Geometry check sheet. Reference: the model listing, model coordinates, mm. Round coordinates to 2 decimals unless told otherwise and drop trailing zeros. Write each loop counter-clockwise with the first axis right and the second up, starting at its lowest first coordinate (ties: lowest second). Pieces come first, ordered by that corner, then holes. Notation, with made-up numbers: (36.25, 69) - (84.25, 69) arc R8 ccw to (84.25, 81) - close; hole circle Ø3 at (69.25, -38.75). An arc over 180 degrees is marked (long way). Return JSON: item names as keys, results as strings.
```python
from build123d import *

# Parameters (mm, degrees)
SKETCH1_W                                  = 63.5
SKETCH1_H                                  = 30.48
BOSS_EXTRUDE1_DEPTH                        = 6.35
TAP_DRILL_FOR_8_32_TAP1_D                  = 3.4544
TAP_DRILL_FOR_8_32_TAP1_DEPTH              = 6.35
TAP_DRILL_FOR_8_32_TAP1_TIP                = 1.037806461
F_6_CLOSE_CLEARANCE_HOLE_COUNTERSINK_D     = 3.6576
F_6_CLOSE_CLEARANCE_HOLE_COUNTERSINK_DEPTH = 6.35
F_8_THROUGH_HOLE_D                         = 5.0546
F_8_THROUGH_HOLE_DEPTH                     = 6.35
F_8_THROUGH_HOLE_TIP                       = 1.518555042


with BuildPart() as part:
    # Sketch1 → Boss-Extrude1 (new body)
    with BuildSketch(Plane(origin=(0, 0, 0), x_dir=(0, 0, -1), z_dir=(1, 0, 0))):
        with Locations((-28.514872299, 20.201128374)):
            Rectangle(SKETCH1_W, SKETCH1_H)
    extrude(amount=BOSS_EXTRUDE1_DEPTH)

    # Tap Drill for #8-32 Tap1
    with Locations(Plane.ZY):
        with Locations((12.639872299, 22.741128374), (44.389872299, 22.741128374)):
            Hole(TAP_DRILL_FOR_8_32_TAP1_D / 2, depth=TAP_DRILL_FOR_8_32_TAP1_DEPTH)
            with Locations((0, 0, -(TAP_DRILL_FOR_8_32_TAP1_DEPTH + TAP_DRILL_FOR_8_32_TAP1_TIP / 2))):  # 118° drill point
                Cone(0, TAP_DRILL_FOR_8_32_TAP1_D / 2, TAP_DRILL_FOR_8_32_TAP1_TIP, mode=Mode.SUBTRACT)

    # #6 Close clearance hole, countersink
    with Locations(Plane.ZY):
        with Locations((9.464872299, 32.266128374), (47.564872299, 32.266128374)):
            Hole(F_6_CLOSE_CLEARANCE_HOLE_COUNTERSINK_D / 2, depth=F_6_CLOSE_CLEARANCE_HOLE_COUNTERSINK_DEPTH)

    # #8 Through hole
    with Locations(Plane.ZY):
        with Locations((53.914872299, 26.974461707)):
            Hole(F_8_THROUGH_HOLE_D / 2, depth=F_8_THROUGH_HOLE_DEPTH)
            with Locations((0, 0, -(F_8_THROUGH_HOLE_DEPTH + F_8_THROUGH_HOLE_TIP / 2))):  # 118° drill point
                Cone(0, F_8_THROUGH_HOLE_D / 2, F_8_THROUGH_HOLE_TIP, mode=Mode.SUBTRACT)


solid = part.part
```
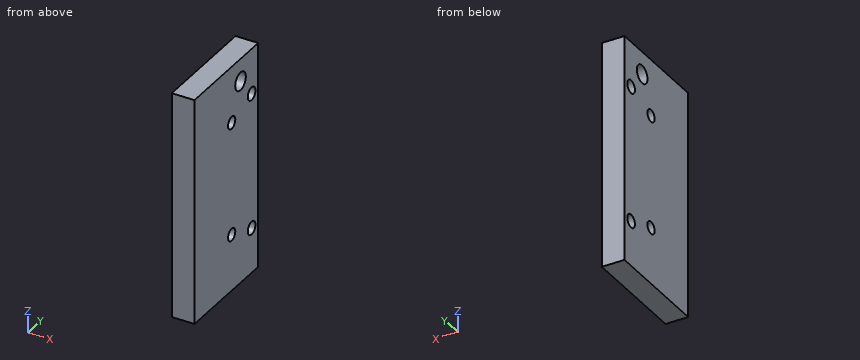
(1) Gauge pin test, flat end, axial feed: pin 1 (6 mm diameter, centred on y = 32.27, z = 9.46, fed in from +X). Record the tip position at first contact, or that the pin passes through.
Response values:
{"pin 1": "stops at x = 6.35"}
(2) Section check B-B, the plane x = 3.25. Enter the section's corners in (y, z).
Response values:
{"outline": "(4.96, -3.24) - (35.44, -3.24) - (35.44, 60.26) - (4.96, 60.26) - close; hole circle Ø3.45 at (22.74, 12.64); hole circle Ø3.45 at (22.74, 44.39); hole circle Ø5.05 at (26.97, 53.91); hole circle Ø3.66 at (32.27, 9.46); hole circle Ø3.66 at (32.27, 47.56)"}
(3) Section check A-A, the plane z = 12. Enter the section's corners in (x, y), plus the area to 3 significant figures.
Response values:
{"outline": "(0, 4.96) - (6.35, 4.96) - (6.35, 21.14) - (0, 21.14) - close; (0, 24.35) - (6.35, 24.35) - (6.35, 35.44) - (0, 35.44) - close", "area": "173 mm^2"}
(4) Material ranges on line 1 along Z through (x, y) = (2.75, 22); line 2 along Z through (x, y) = (4.25, 31); line 3 along Z through (x, y) = (0.5, 28) (3 decimals), recorded low to high. Write a range as [from, to].
Response values:
{"line 1": "z = [-3.24, 11.08], [14.2, 42.83], [45.95, 60.26]", "line 2": "z = [-3.24, 8.15], [10.78, 46.25], [48.88, 60.26]", "line 3": "z = [-3.235, 51.605], [56.225, 60.265]"}
